CAD build for the part. Positions are in the model's coordinates, mm. Give positions to 0.01 mm unless a question says otherwise; leave off trailing zeros. Order: outer loops, then holes, each group sorted by start corner. A loop starts at its lowest first (then second) coordinate and runs counter-clockwise, first axis right, second up. Notation, with made-up numbers: (-24, -36.5) -> (1, -36.5) arc R26 cw to (1, -15.5) -> close; hole circle Ø10 at (68.25, -34.5). An arc over 180 degrees is marked (long way). Use one line per item in the form item = value. Start each with the question number.
1) Cut at A-A, the plane x = 0. Give the cut face in (y, z), and give its area (3 significant figures).
2) Probe line 1 (X direction, y = -0.5, z = 250); line 2 (Z direction, x = -0.5, y = 7.25). List the from-to ranges inside material, lowest first.
3) Drop flat-ended pins along their axis: P1, Ø1.3, axis at y = 5, z = 148.5, coming from the +X side; P2, Ø1.9, axis at y = 6.5, z = 285.5, coming from the +X side; P3, Ø1.8, axis at y = 5, z = 148.5, coming from the -X side. Give the stop position or say it passes through.
4) Cut at C-C, the plane z = 263. Give the cut face in (x, y).
5) Cut at B-B, the plane z = 140.5. Give the cut face in (x, y).
from build123d import *

# Parameters (mm, degrees)
SKETCH_1_R          = 6
EXTRUDE_1_DEPTH     = 300
SKETCH_2_W          = 4
SKETCH_2_H          = 5.416856643
EXTRUDE_2_DEPTH     = 22.91
CUT_EXTRUDE_START   = 6
CUT_EXTRUDE_1_DEPTH = 2


with BuildPart() as part:
    # 草图1 → 凸台-拉伸1 (new body)
    with BuildSketch(Plane.XY):
        Circle(SKETCH_1_R)
    extrude(amount=EXTRUDE_1_DEPTH)

    # 草图2 → 凸台-拉伸2 (add)
    with BuildSketch(Plane.XY.offset(300)):
        with Locations((0, 5.291571679)):
            Rectangle(SKETCH_2_W, SKETCH_2_H)
    extrude(amount=-EXTRUDE_2_DEPTH)

    # 草图3 → 切除-拉伸1 (cut)
    with BuildSketch(Plane(origin=(0, 0, 0), x_dir=(1, 0, 0), z_dir=(0, 1, 0)).offset(CUT_EXTRUDE_START)):
        with BuildLine():
            Line((2, -125.29796429), (2, -179.002027522))
            ThreePointArc((2, -179.002027522), (0, -181.002027522), (-2, -179.002027522))
            Line((-2, -179.002027522), (-2, -125.29796429))
            ThreePointArc((-2, -125.29796429), (0, -123.29796429), (2, -125.29796429))
        make_face()
    extrude(amount=-CUT_EXTRUDE_1_DEPTH, mode=Mode.SUBTRACT)


solid = part.part
Result:
q1.outline = (-6, 0) -> (6, 0) -> (6, 123.3) -> (4, 123.3) -> (4, 181) -> (6, 181) -> (6, 277.09) -> (8, 277.09) -> (8, 300) -> (-6, 300) -> close
q1.area = 3,530 mm²
q2.line_1 = -5.98 to 5.98
q2.line_2 = 277.09 to 300
q3.P1 = 4.13
q3.P2 = 2.28
q3.P3 = -4.38
q4.outline = circle Ø12 at (0, 0)
q5.outline = (-2, 4) -> (-2, 5.66) arc R6 ccw (long way) to (2, 5.66) -> (2, 4) -> close
